Answer from the drawing. Dimensions are ordinates in mm from the lowest x, y and z of the part. A direction names the side the tool comes from. Coordinates: 2 decimals unless noted, no trailing zeros. Write each loop counter-clockwise with the first axis right and the second up, starting at its lowest first coordinate (ties: lowest second). Pieces come first, ordered by that corner, then holes. Notation, with made-up numbers: (-18, 74) -> (-14, 74) arc R20 ccw to (-14, 85) -> close; hole circle Ø10 at (72.25, 84.5). An arc over 180 degrees is marked (long way). Return JSON: item names as keys, results as strings.
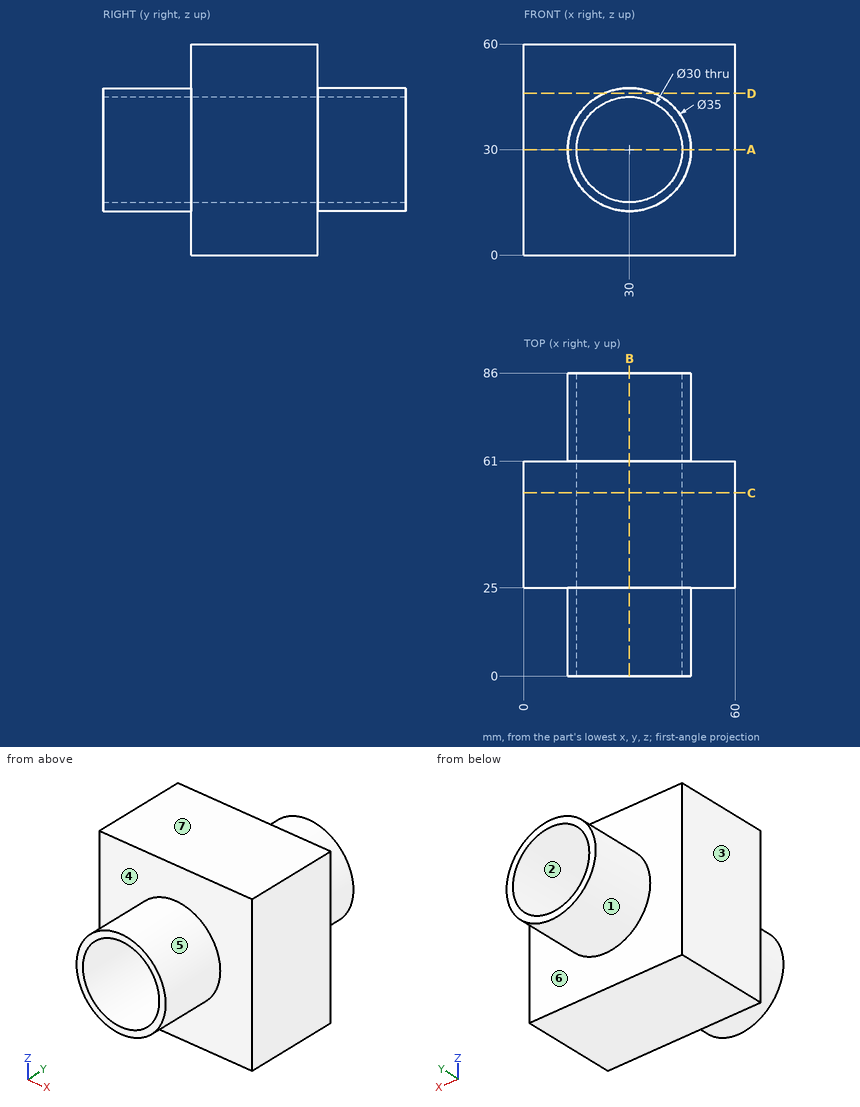
1. The part is cut by section B-B (x = 30). Determine the outline of the cut face in (y, z).
Taken from the geometry:
{"outline": "(0, 12.5) -> (25, 12.5) -> (25, 0) -> (61, 0) -> (61, 12.5) -> (86, 12.5) -> (86, 15) -> (0, 15) -> close; (0, 45) -> (86, 45) -> (86, 47.5) -> (61, 47.5) -> (61, 60) -> (25, 60) -> (25, 47.5) -> (0, 47.5) -> close"}
2. The part is cut by section C-C (y = 52). Determine the outline of the cut face in (x, z).
Taken from the geometry:
{"outline": "(0, 0) -> (60, 0) -> (60, 60) -> (0, 60) -> close; hole circle Ø30 at (30, 30)"}
3. Flat-ended cylindrical pins translate along their axes: pin 1 Ø1.5 at (x, y) = (37.5, 59) entering from -Z; pin 2 Ø2 at (x, z) = (39.5, 54) entering from +Y; pin 3 Ø18 at (x, z) = (30, 30) entering from +Y. Find the tip coordinate at first contact, or state that the pin passes through.
Taken from the geometry:
{"pin 1": "stops at z = 0", "pin 2": "stops at y = 61", "pin 3": "passes through"}
4. The part is cut by section A-A (z = 30). Determine the outline of the cut face in (x, y).
Taken from the geometry:
{"outline": "(0, 25) -> (12.5, 25) -> (12.5, 0) -> (15, 0) -> (15, 86) -> (12.5, 86) -> (12.5, 61) -> (0, 61) -> close; (45, 0) -> (47.5, 0) -> (47.5, 25) -> (60, 25) -> (60, 61) -> (47.5, 61) -> (47.5, 86) -> (45, 86) -> close"}
5. For a pull along X with two mould halves and no side action, classify the marked faces 1, 2, 3 and 4 as +X half, -X half, draft (parallel to the pull), parting line (faces both ways), or undercut.
Taken from the geometry:
{"face 1": "parting line", "face 2": "undercut", "face 3": "-X half", "face 4": "draft"}
6. A tool of negligible diameter and unlimited length cuts with its end or side. For the marked faces 5, 6 and 7, from which of +Z, -Z, +X, -X, +Y, -Y can it reach the whole face along a straight path? Write none if from no direction.
Taken from the geometry:
{"face 5": "-Y", "face 6": "+Y", "face 7": "+Z, +X, -X, +Y, -Y"}
7. Consider L1, parallel to Z at x = 30, y = 18; L2, parallel to Z at x = 30, y = 47; L3, parallel to Y at x = 27, z = 56. Determine where each line is inside the solid, lowest interval first.
Taken from the geometry:
{"L1": "z = 12.5 to 15, 45 to 47.5", "L2": "z = 0 to 15, 45 to 60", "L3": "y = 25 to 61"}
8. The part is cut by section D-D (z = 46). Determine the outline of the cut face in (x, y).
Taken from the geometry:
{"outline": "(0, 25) -> (22.91, 25) -> (22.91, 0) -> (37.09, 0) -> (37.09, 25) -> (60, 25) -> (60, 61) -> (37.09, 61) -> (37.09, 86) -> (22.91, 86) -> (22.91, 61) -> (0, 61) -> close"}
